Geometry check sheet. Reference: drawing and pictorial views, mm from the part's lowest x, y, z. A direction names the side the tool comes from. Round coordinates to 2 decimals unless told otherwise and drop trailing zeros. Loops run counter-clockwise (first coordinate to the right, second up) from the corner with the lowest first, then second, coordinate; pieces in that order, holes last. Notation, with made-up numbers: M 45,47.25 L 50,47.25 A24 ccw 50,81.25 Z; hole C 78.25,-40 d2. An arc over 180 degrees is marked long. One line per question, with ' | ' between items. Start each with the question number.
(1) Go/stop test with flat-tipped pins: P1, Ø1.5, axis at y = 22, z = 1.5, coming from the +X side; P2, Ø0.9, axis at x = 12, z = 2, coming from the +Y side; P3, Ø0.9, axis at x = 14.5, z = 1.5, coming from the -Y side; P4, Ø2, axis at x = 6, y = 16.5, coming from the -Z side. Record where each tip stops, or that it passes through.
(2) Section check B-B (x = 6). Record the boundary of the cut face in (y, z).
(3) Section check C-C (y = 1.5). Record the boundary of the cut face in (x, z), and give its area (3 significant figures).
(4) Section check D-D (x = 18). Record the boundary of the cut face in (y, z), and give its area (3 significant figures).
(5) Section check A-A (z = 2.1). Record the boundary of the cut face in (x, y), and give its area (3 significant figures).
(6) Draft check along Y on the marked faces 4, 5 and 6. Enter one of: +Y half, -Y half, draft (parallel to the pull), parting line (faces both ways), or undercut.
(7) Tool access check on the marked faces 1, 2 and 3. Record the directions out of +Z, -Z, +X, -X, +Y, -Y that give a thin tool (end or side, any length) a straight path to the whole face; none if there is none.
(8) Thickness scan on probe 1 along Y at (x, z) = (2.45, 1.5); probe 2 along Y at (x, z) = (5, 1.2); probe 3 along X at (y, z) = (1.5, 0.4). Record the ranges inside material, lowest first. Write a range as [from, to].
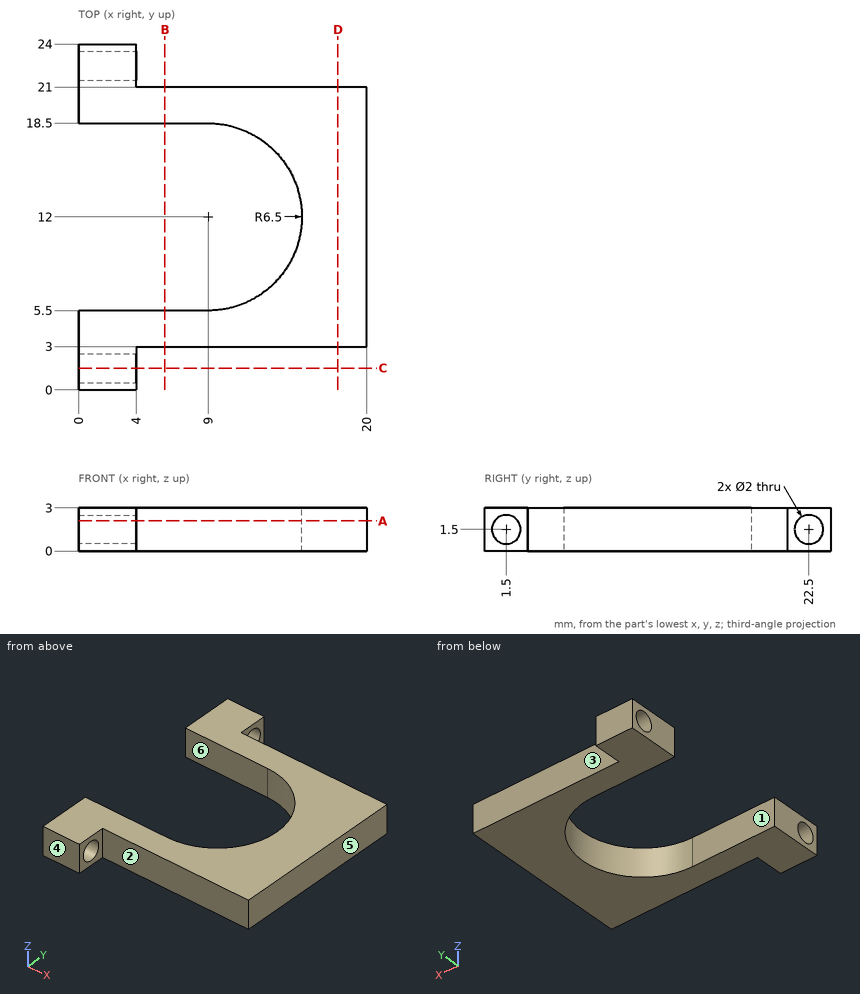
The answers:
1) P1: x = 4 | P2: y = 21 | P3: y = 3 | P4: through
2) outline: M 3,0 L 5.5,0 L 5.5,3 L 3,3 Z; M 18.5,0 L 21,0 L 21,3 L 18.5,3 Z
3) outline: M 0,0 L 4,0 L 4,0.5 L 0,0.5 Z; M 0,2.5 L 4,2.5 L 4,3 L 0,3 Z | area: 4.00 mm²
4) outline: M 3,0 L 21,0 L 21,3 L 3,3 Z | area: 54.0 mm²
5) outline: M 0,0 L 4,0 L 4,0.7 L 0,0.7 Z; M 0,2.3 L 4,2.3 L 4,3 L 20,3 L 20,21 L 4,21 L 4,21.7 L 0,21.7 L 0,18.5 L 9,18.5 A6.5 cw 9,5.5 L 0,5.5 Z; M 0,23.3 L 4,23.3 L 4,24 L 0,24 Z | area: 188 mm²
6) face 4: -Y half | face 5: draft | face 6: undercut
7) face 1: +Z, -Z, -X | face 2: +Z, -Z, +X, -Y | face 3: +Z, -Z, +X, +Y
8) probe 1: [0, 0.5], [2.5, 5.5], [18.5, 21.5], [23.5, 24] | probe 2: [3, 5.5], [18.5, 21] | probe 3: [0, 4]
